Can you work these out from the model? Positions are in its coordinate system, mm. Face numbers are marked on the shaded views. A direction names the side the tool comes from. Give positions to 0.01 mm unless a question says otherwise; leave off trailing zeros. Write each loop counter-clockwise with the first axis right and the second up, starting at its lowest first coordinate (ties: lowest second). Pieces come first, ordered by that corner, then holes.
1. If I drill on probe 1 along Y at (x, z) = (-9, -20); probe 2 along Y at (x, z) = (29, -19); probe 3 along Z at (x, y) = (60.5, 58), over which ranges is the centre line in solid material (lowest first)?
2. On a 3-axis mill with a long thin cutter (end or side, diameter ignored), from which of +Z, -Z, +X, -X, +Y, -Y can I reach the whole of each face in a straight line? I mean the marked faces 1 and 2. Say none if no direction works.
3. Suppose I cut it at A-A (z = -20). Please give me the cut outline in (x, y), and give its area (3 significant figures).
4. I'm going to push flat-ended pins straight in: pin 1 (2 mm diameter, centred on x = -72, y = -60.5, fed in from -Z); pin 2 (4 mm diameter, centred on x = -13.5, z = -4.5, fed in from -Y); pin 3 (4 mm diameter, centred on y = 65, z = -9, fed in from -X). Where does each tip first touch, or does it pass through?
5. Thinking about a two-plate mould opening in Y: for the marked faces 3, 4 and 5, which applies, pulls with the +Y half, pulls with the -Y half, needs draft (parallel to the pull), parting line crosses it, or undercut?
6. Suppose I cut it at D-D (x = 15). Please give me the cut outline in (y, z), and give its area (3 significant figures).
7. Suppose I cut it at B-B (y = 80). Please give me the cut outline in (x, z).
8. Suppose I cut it at C-C (z = -35.5). Please give me the cut outline in (x, y), and give its area (3 significant figures).
Autodesk Inventor part; units mm, degrees
ref_plane "YZ Plane" through (0, 0, 0) normal (1, 0, 0) x (0, 1, 0)
ref_plane "XZ Plane" through (0, 0, 0) normal (0, 1, 0) x (-1, 0, 0)
ref_plane "XY Plane" through (0, 0, 0) normal (0, 0, 1) x (1, 0, 0)
sketch "Sketch1" plane through (0, 0, 0) normal (0, 0, 1) x (1, 0, 0)
  line L0 (150, -133) -> (-150, -133)
  line L1 (-150, -133) -> (-150, 133)
  line L2 (-150, 133) -> (150, 133)
  line L3 (150, 133) -> (150, -133)
  line L4 (0, 0) -> (0, 81.3474)
  line L5 (0, 0) -> (80.8517, 0)
  point P0 (0, 133)
  point P1 (150, 0)
  dimension "d0" = 300
  dimension "d1" = 266
extrude "Extrusion1" add sketch "Sketch1" along normal blind 10
sketch "Sketch2" plane through (0, 0, 0) normal (0, 0, -1) x (-1, 0, 0)
  line L0 (35, -35) -> (-35, -35)
  line L1 (-35, -35) -> (-35, 35)
  line L2 (-35, 35) -> (35, 35)
  line L3 (35, 35) -> (35, -35)
  line L4 (0, 0) -> (0, 15.9444)
  line L5 (0, 0) -> (16.1389, 0)
  line L6 (35, -95) -> (-35, -95)
  line L7 (-35, -95) -> (-35, -65)
  line L8 (-35, -65) -> (35, -65)
  line L9 (35, -65) -> (35, -95)
  line L10 (35, 65) -> (-35, 65)
  line L11 (-35, 65) -> (-35, 95)
  line L12 (-35, 95) -> (35, 95)
  line L13 (35, 95) -> (35, 65)
  point P0 (0, 35)
  point P1 (35, 0)
  dimension "d4" = 70
  dimension "d7" = 70
  dimension "d8" = 30
  dimension "d9" = 30
  dimension "d10" = 30
  dimension "d11" = 30
extrude "Extrusion2" add sketch "Sketch2" along normal blind 14 contours L0 L1 L2 L3
extrude "Extrusion3" add sketch "Sketch2" along normal blind 40 contours L6 L7 L8 L9 | L10 L11 L12 L13
sketch "Sketch3" plane through (-35, 65, 0) normal (-1, 0, 0) x (0, 0, 1)
  line L0 (0, 30) -> (-40, 30)
  line L1 (-40, 0) -> (-40, 30)
  circle A0 centre (-20, 15) radius 8
  point P0 (0, -65)
  dimension "d14" = 16
  dimension "d15" = 15
  dimension "d16" = 20
extrude "Extrusion4" cut sketch "Sketch3" against normal through all
sketch "Sketch4" plane through (-35, -95, 0) normal (-1, 0, 0) x (0, 0, 1)
  line L0 (0, 30) -> (-40, 30)
  line L1 (-40, 0) -> (-40, 30)
  circle A0 centre (-20, 15) radius 8
  point P0 (0, 95)
  dimension "d19" = 16
  dimension "d20" = 15
  dimension "d21" = 20
extrude "Extrusion5" cut sketch "Sketch4" against normal through all
thread "Thread1"
thread "Thread2"
properties part number "Plate" material "Wood (Walnut)"
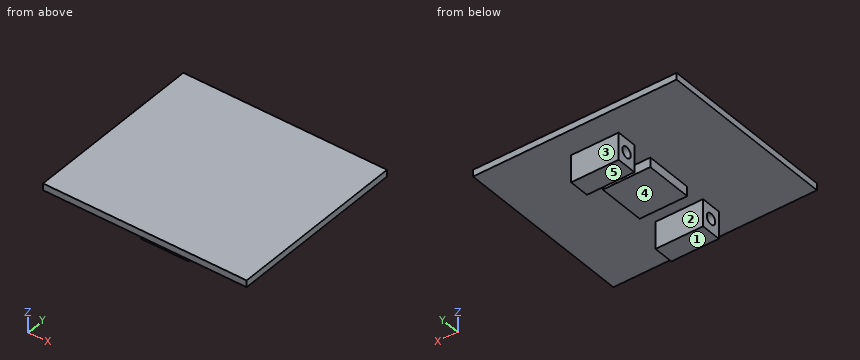
Checks:
1. probe 1: y = -95 to -88, -72 to -65, 65 to 72, 88 to 95
1. probe 2: y = -95 to -87.94, -72.06 to -65, 65 to 72.06, 87.94 to 95
1. probe 3: z = 0 to 10
2. face 1: -Z, +X, -X, +Y, -Y
2. face 2: -Z, +X, -X
3. outline: (-35, -95) - (35, -95) - (35, -88) - (-35, -88) - close; (-35, -72) - (35, -72) - (35, -65) - (-35, -65) - close; (-35, 65) - (35, 65) - (35, 72) - (-35, 72) - close; (-35, 88) - (35, 88) - (35, 95) - (-35, 95) - close
3. area: 1,960 mm2
4. pin 1: stops at z = 0
4. pin 2: stops at y = -95
4. pin 3: stops at x = -35
5. face 3: pulls with the +Y half
5. face 4: undercut
5. face 5: needs draft
6. outline: (-133, 0) - (-95, 0) - (-95, -40) - (-65, -40) - (-65, 0) - (-35, 0) - (-35, -14) - (35, -14) - (35, 0) - (65, 0) - (65, -40) - (95, -40) - (95, 0) - (133, 0) - (133, 10) - (-133, 10) - close; hole circle Ø16 at (-80, -20); hole circle Ø16 at (80, -20)
6. area: 5,640 mm2
7. outline: (-150, 0) - (-35, 0) - (-35, -12) - (35, -12) - (35, 0) - (150, 0) - (150, 10) - (-150, 10) - close; (-35, -40) - (35, -40) - (35, -28) - (-35, -28) - close
8. outline: (-35, -95) - (35, -95) - (35, -65) - (-35, -65) - close; (-35, 65) - (35, 65) - (35, 95) - (-35, 95) - close
8. area: 4,200 mm2
